Design review of the part built by this model. Coordinates are the model's own, in mm. Face numbers are marked on the shaded views. A direction names the side the tool comes from. Coordinates: 2 decimals unless noted, no trailing zeros. Order: outer loops, then holes, each group sorted by start corner. A loop starts at its lowest first (then second) coordinate and runs counter-clockwise, first axis right, second up. Notation, with made-up numbers: M 55,27.25 L 68,27.25 A17 ccw 68,34.25 Z; hole C 77,-23.5 d1. An arc over 180 degrees is marked long. Answer in a Markdown table with one row per item.
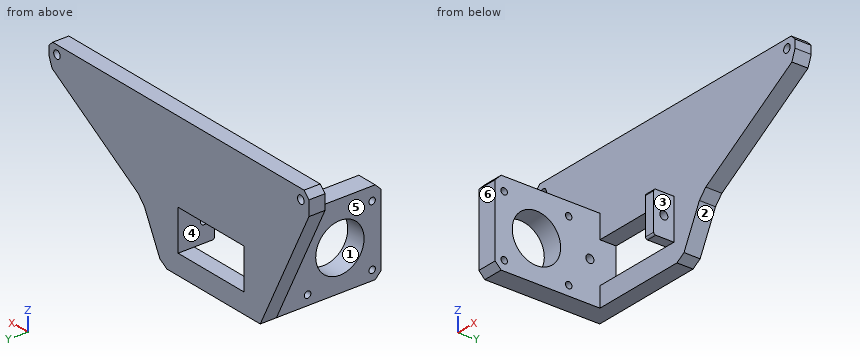
from build123d import *

# Parameters (mm, degrees)
CROQUIS1_R              = 2
CROQUIS1_W              = 53.3
CROQUIS1_H              = 20.15
SALIENTE_EXTRUIR1_DEPTH = 8
CROQUIS2_W              = 7.991381739
CROQUIS2_H              = 20.15
SALIENTE_EXTRUIR2_DEPTH = 60
CROQUIS2_4_W            = 5
CROQUIS2_4_H            = 20.15
SALIENTE_EXTRUIR3_DEPTH = 18
CROQUIS3_R              = 2
CORTAR_EXTRUIR1_DEPTH   = 107
CROQUIS3_3_R            = 2
CORTAR_EXTRUIR2_DEPTH   = 8
CROQUIS5_R              = 1.6
CROQUIS5_R_2            = 12
CORTAR_EXTRUIR3_DEPTH   = 59


with BuildPart() as part:
    # Croquis1 → Saliente-Extruir1 (new body)
    with BuildSketch(Plane(origin=(0, 0, 0), x_dir=(1, 0, 0), z_dir=(0, 1, 0))):
        Polygon((154, 0), (156.396068252, 2.352828169), (156.396068252, 6.352828169), (154.446539538, 11.574918968), (101.665094886, 44.198861104), (97.772883017, 48.458390041), (88.347282669, 67.313746258), (84.009081739, 69.99516616), (26.841381739, 69.99516616), (-2.995601596, 10.334082852), (-2.995601596, 3.004082852), (0, 0), align=None)
        with Locations((2, 5)):
            Circle(CROQUIS1_R, mode=Mode.SUBTRACT)
        with Locations((151.397935499, 4.352828169)):
            Circle(CROQUIS1_R, mode=Mode.SUBTRACT)
        with Locations((55.5, 50.075)):
            Rectangle(CROQUIS1_W, CROQUIS1_H, mode=Mode.SUBTRACT)
    extrude(amount=SALIENTE_EXTRUIR1_DEPTH)

    # Croquis2 → Saliente-Extruir2 (add)
    with BuildSketch(Plane(origin=(0, 8, 0), x_dir=(1, 0, 0), z_dir=(0, 1, 0))):
        Polygon((36.841381739, 69.99516616), (26.841381739, 69.99516616), (26.841381739, 28.39516616), (36.841381739, 28.39516616), (36.841381739, 40), (28.85, 40), (28.85, 60.15), (36.841381739, 60.15), align=None)
        with Locations((32.84569087, 50.075)):
            Rectangle(CROQUIS2_W, CROQUIS2_H)
    extrude(amount=-SALIENTE_EXTRUIR2_DEPTH)

    # Croquis2_4 → Saliente-Extruir3 (add)
    with BuildSketch(Plane(origin=(0, 8, 0), x_dir=(1, 0, 0), z_dir=(0, 1, 0))):
        with Locations((79.65, 50.075)):
            Rectangle(CROQUIS2_4_W, CROQUIS2_4_H)
    extrude(amount=-SALIENTE_EXTRUIR3_DEPTH)

    # Croquis3 → Cortar-Extruir1 (cut)
    with BuildSketch(Plane(origin=(82.15, 0, 0), x_dir=(0, 0, -1), z_dir=(1, 0, 0))):
        with Locations((50.075, -5)):
            Circle(CROQUIS3_R)
    extrude(amount=-CORTAR_EXTRUIR1_DEPTH, mode=Mode.SUBTRACT)

    # Croquis3_3 → Cortar-Extruir2 (cut)
    with BuildSketch(Plane(origin=(82.15, 0, 0), x_dir=(0, 0, -1), z_dir=(1, 0, 0))):
        with Locations((50.075, -5)):
            Circle(CROQUIS3_3_R)
        with BuildLine():
            Line((59.15, -10), (60.15, -10))
            Line((60.15, -10), (60.15, -9))
            ThreePointArc((60.15, -9), (59.857106781, -9.707106781), (59.15, -10))
        make_face()
        with BuildLine():
            Line((40, -10), (40, -9))
            ThreePointArc((40, -9), (40.292893219, -9.707106781), (41, -10))
            Line((41, -10), (40, -10))
        make_face()
    extrude(amount=-CORTAR_EXTRUIR2_DEPTH, mode=Mode.SUBTRACT)

    # Croquis5 → Cortar-Extruir3 (cut)
    with BuildSketch(Plane(origin=(36.841381739, 0, 0), x_dir=(0, 0, -1), z_dir=(1, 0, 0))):
        with Locations((65.165, -15.5)):
            Circle(CROQUIS5_R)
        with Locations((50.075, -31.5)):
            Circle(CROQUIS5_R_2)
        with Locations((65.165, -47.5)):
            Circle(CROQUIS5_R)
        with Locations((34.985, -15.5)):
            Circle(CROQUIS5_R)
        with Locations((34.985, -47.5)):
            Circle(CROQUIS5_R)
        Polygon((28.39516616, -52), (28.39516616, -49), (31.39516616, -52), align=None)
        Polygon((69.99516616, -52), (69.99516616, -49), (66.99516616, -52), align=None)
    extrude(amount=-CORTAR_EXTRUIR3_DEPTH, mode=Mode.SUBTRACT)


solid = part.part
(1) Add section B-B, the plane y = -5. Give the boundary of the cut face in (x, z) (3 decimals).
Return value:
| item | result |
|---|---|
| outline | M 26.841,-69.995 L 36.841,-69.995 L 36.841,-52.075 L 26.841,-52.075 Z; M 26.841,-48.075 L 36.841,-48.075 L 36.841,-28.395 L 26.841,-28.395 Z; M 77.15,-60.15 L 82.15,-60.15 L 82.15,-52.075 L 77.15,-52.075 Z; M 77.15,-48.075 L 82.15,-48.075 L 82.15,-40 L 77.15,-40 Z |
(2) Add section D-D, the plane y = -31.5. Give the boundary of the cut face in (x, z) (3 decimals).
Return value:
| item | result |
|---|---|
| outline | M 26.841,-69.995 L 36.841,-69.995 L 36.841,-62.075 L 26.841,-62.075 Z; M 26.841,-38.075 L 36.841,-38.075 L 36.841,-28.395 L 26.841,-28.395 Z |
(3) Add section C-C, the plane x = 69.5. Give the boundary of the cut face in (y, z), and give its area (3 significant figures).
Return value:
| item | result |
|---|---|
| outline | M 0,-70 L 8,-70 L 8,-60.15 L 0,-60.15 Z; M 0,-40 L 8,-40 L 8,0 L 0,0 Z |
| area | 399 mm2 |
(4) Add section A-A, the plane y = -47.5. Give the boundary of the cut face in (x, z) (3 decimals), and give its area (3 significant figures).
Return value:
| item | result |
|---|---|
| outline | M 26.841,-69.995 L 36.841,-69.995 L 36.841,-66.765 L 26.841,-66.765 Z; M 26.841,-63.565 L 36.841,-63.565 L 36.841,-36.585 L 26.841,-36.585 Z; M 26.841,-33.385 L 36.841,-33.385 L 36.841,-28.395 L 26.841,-28.395 Z |
| area | 352 mm2 |
(5) For the marked faces 4, 5 and 6, list the 3-axis set-ups (+Z, -Z, +X, -X, +Y, -Y) from which the entire face can be reached by the end or side of a thin tool; tool diameter is ignored.
Return value:
| item | result |
|---|---|
| face 4 | +Y, -Y |
| face 5 | +Z, -Z, -X, -Y |
| face 6 | +Z, -Z, +X, -X, -Y |
(6) Insertion check: pin 1 Ø1.5 at (y, z) = (-24, -32) entering from +X; pin 2 Ø10 at (x, z) = (55.5, -21.5) entering from -Y; pin 3 Ø8 at (x, y) = (34.5, -20.5) entering from +Z. Each pin has a flat end and moves straight along its axis. Give the tip position at first contact, or say it passes through.
Return value:
| item | result |
|---|---|
| pin 1 | stops at x = 36.84 |
| pin 2 | stops at y = 0 |
| pin 3 | stops at z = -28.4 |
(7) For line 1 along Z through (x, y) = (33, -15); line 2 along Y through (x, z) = (84, -59); line 3 along X through (y, z) = (-6, -60.5), list the stretches that pass through material, from the lowest coordinate up. Write a range as from..to.
Return value:
| item | result |
|---|---|
| line 1 | z = -70..-66.68, -63.65..-36.5, -33.47..-28.4 |
| line 2 | y = 0..8 |
| line 3 | x = 26.84..36.84 |
(8) Draft analysis for pull direction Z (two halves, no side actions). For the marked faces 1, 2 and 3, state which applies: pulls with the +Z half, pulls with the -Z half, needs draft (parallel to the pull), parting line crosses it, or undercut.
Return value:
| item | result |
|---|---|
| face 1 | undercut |
| face 2 | pulls with the -Z half |
| face 3 | needs draft |
